Input: part model. Units: mm. Frame: model coordinates. Coordinates: 2 decimals unless noted, no trailing zeros. Write each loop counter-clockwise with the first axis right and the second up, starting at its lowest first coordinate (ties: lowest second). Pieces come first, ordered by that corner, then holes. Notation, with made-up numbers: (67.5, -39.5) - (121.5, -39.5) arc R14 cw to (121.5, -16.5) - close; hole circle Ø8 at (52, 53). An arc over 180 degrees is marked (long way). One line per question, with ' | ' between items. Start each with the question number.
1) Section query A-A on z = 0. Return loops of the section in (x, y).
2) Section query C-C on y = 3. Return loops of the section in (x, z) (3 decimals), and give its area (3 significant figures).
3) Line query: line 1 (X direction, y = 4, z = -20); line 2 (X direction, y = 3.75, z = -1); line 3 (X direction, y = 2.25, z = -21). Output: solid intervals per line, ascending.
4) Section query B-B on x = 8. Return loops of the section in (y, z).
```python
from build123d import *

# Parameters (mm, degrees)
SKETCH1_W           = 123.698
SKETCH1_H           = 76.454
BOSS_EXTRUDE1_DEPTH = 6.35
SKETCH6_R           = 19.05
SKETCH6_R_2         = 3.81
CUT_EXTRUDE5_DEPTH  = 73.985785123
FILLET1_R           = 0.254


with BuildPart() as part:
    # Sketch1 → Boss-Extrude1 (new body)
    with BuildSketch(Plane(origin=(0, 0, 0), x_dir=(1, 0, 0), z_dir=(0, 1, 0))):
        Rectangle(SKETCH1_W, SKETCH1_H)
    extrude(amount=BOSS_EXTRUDE1_DEPTH)

    # Sketch6 → Cut-Extrude5 (cut, through all)
    with BuildSketch(Plane(origin=(0, 6.35, 0), x_dir=(1, 0, 0), z_dir=(0, 1, 0))):
        with Locations(Location((-3.633226289, 0, 0), (0, 0, 270))):
            Circle(SKETCH6_R)
        with Locations(Location((16.482547422, 20.115773711, 0), (0, 0, 270))):
            Circle(SKETCH6_R_2)
        with Locations(Location((-23.749, 20.115773711, 0), (0, 0, 270))):
            Circle(SKETCH6_R_2)
        with Locations(Location((-23.749, -20.115773711, 0), (0, 0, 270))):
            Circle(SKETCH6_R_2)
        with Locations(Location((16.482547422, -20.115773711, 0), (0, 0, 270))):
            Circle(SKETCH6_R_2)
        with Locations(Location((-49.149, 15.875, 0), (0, 0, 270))):
            Circle(SKETCH6_R_2)
        with Locations(Location((-49.149, -15.875, 0), (0, 0, 270))):
            Circle(SKETCH6_R_2)
    extrude(amount=-CUT_EXTRUDE5_DEPTH, mode=Mode.SUBTRACT)

    # Fillet1
    fillet1_edges = [part.edges().sort_by_distance(p)[0] for p in [
        (61.849, 3.175, 38.227),
        (-61.849, 3.175, 38.227),
        (-61.849, 3.175, -38.227),
        (61.849, 3.175, -38.227),
    ]]
    fillet(fillet1_edges, radius=FILLET1_R)


solid = part.part
```
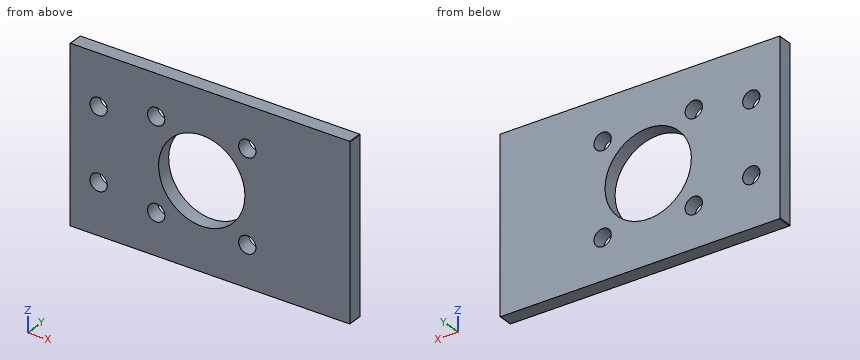
Answer key:
1) outline: (-61.85, 0) - (-22.68, 0) - (-22.68, 6.35) - (-61.85, 6.35) - close; (15.42, 0) - (61.85, 0) - (61.85, 6.35) - (15.42, 6.35) - close
2) outline: (-61.849, -37.973) arc R0.254 ccw to (-61.595, -38.227) - (61.595, -38.227) arc R0.254 ccw to (61.849, -37.973) - (61.849, 37.973) arc R0.254 ccw to (61.595, 38.227) - (-61.595, 38.227) arc R0.254 ccw to (-61.849, 37.973) - close; hole circle Ø7.62 at (-49.149, -15.875); hole circle Ø7.62 at (-49.149, 15.875); hole circle Ø7.62 at (-23.749, -20.116); hole circle Ø7.62 at (-23.749, 20.116); hole circle Ø38.1 at (-3.633, 0); hole circle Ø7.62 at (16.483, -20.116); hole circle Ø7.62 at (16.483, 20.116) | area: 8,040 mm²
3) line 1: -61.85 to -27.56, -19.94 to 12.67, 20.29 to 61.85 | line 2: -61.85 to -22.66, 15.39 to 61.85 | line 3: -61.85 to -27.45, -20.04 to 12.78, 20.19 to 61.85
4) outline: (0, -38.23) - (6.35, -38.23) - (6.35, -15.09) - (0, -15.09) - close; (0, 15.09) - (6.35, 15.09) - (6.35, 38.23) - (0, 38.23) - close
